Verification items for the finished model (mm, model axes). Face numbers are marked on the shaded views. A direction names the side the tool comes from. Give positions to 0.01 mm unless a question says otherwise; leave off trailing zeros. Loops run counter-clockwise (first coordinate to the right, second up) from the corner with the lowest first, then second, coordinate; pieces in that order, holes last. Notation, with made-up numbers: (71, -7.75) -> (117, -7.75) arc R15 cw to (117, 5.25) -> close; hole circle Ø6 at (61, -12). An arc over 180 degrees is marked (long way). Use one line per item in the form item = value. Start each with the question number.
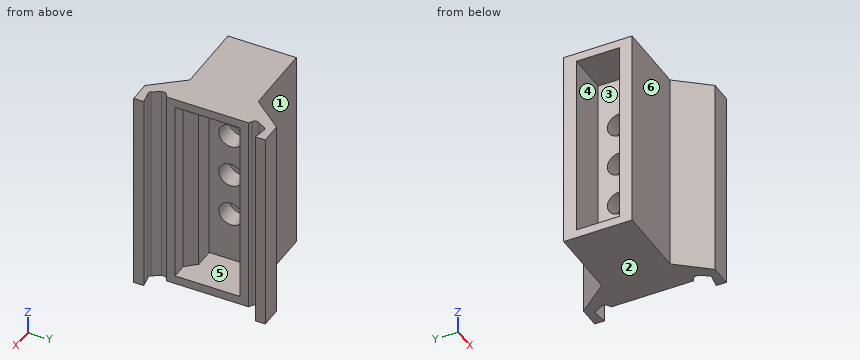
from build123d import *

# Parameters (mm, degrees)
BOSS_EXTRU_1_DEPTH      = 11.98
BOSS_EXTRU_1_DEPTH_BACK = 11.98
BOSS_EXTRU_2_DEPTH      = 1
ESQUISSE3_R             = 1.4
ENL_V_MAT_EXTRU_1_DEPTH = 16.868545408


with BuildPart() as part:
    # Esquisse1 → Boss.-Extru.1 (new, two sides: drawn at the far end of the back side and taken through both)
    with BuildSketch(Plane.XY.offset(-BOSS_EXTRU_1_DEPTH_BACK)):
        with BuildLine():
            Line((0, 4), (0, 2.5))
            Line((0, 2.5), (4.8, 2.5))
            Line((4.8, 2.5), (4.8, -2.5))
            Line((4.8, -2.5), (0, -2.5))
            Line((0, -2.5), (0, -4))
            Line((0, -4), (8.500076, -4))
            Line((8.500076, -4), (11.500006965, -7.699978353))
            Line((11.500006965, -7.699978353), (14, -7.699978353))
            Line((14, -7.699978353), (14, -6.524983133))
            Line((14, -6.524983133), (12.498521064, -6.789609096))
            ThreePointArc((12.498521064, -6.789609096), (12.319554673, -6.766083995), (12.186482634, -6.644124034))
            Line((12.186482634, -6.644124034), (11.641375242, -5.699594361))
            ThreePointArc((11.641375242, -5.699594361), (11.590815941, -5.322605229), (11.820116831, -5.019128457))
            Line((11.820116831, -5.019128457), (12.19995, -4.799870197))
            Line((12.19995, -4.799870197), (12.19995, -3.799987301))
            Line((12.19995, -3.799987301), (10.399918669, -3.799987301))
            Line((10.399918669, -3.799987301), (9.3, -2.549913972))
            Line((9.3, -2.549913972), (7, -2.549913972))
            Line((7, -2.549913972), (7, 2.550086028))
            Line((7, 2.550086028), (9.3, 2.550086028))
            Line((9.3, 2.550086028), (10.399918669, 3.800106202))
            Line((10.399918669, 3.800106202), (12.19995, 3.800106202))
            Line((12.19995, 3.800106202), (12.19995, 4.800033133))
            Line((12.19995, 4.800033133), (11.824382637, 5.01686254))
            ThreePointArc((11.824382637, 5.01686254), (11.591449393, 5.320453932), (11.641389736, 5.699837105))
            Line((11.641389736, 5.699837105), (12.186568343, 6.644209348))
            ThreePointArc((12.186568343, 6.644209348), (12.319573629, 6.766106706), (12.4984419, 6.789676051))
            Line((12.4984419, 6.789676051), (14, 6.524983133))
            Line((14, 6.524983133), (14, 7.700021647))
            Line((14, 7.700021647), (11.499988165, 7.700021647))
            Line((11.499988165, 7.700021647), (8.500082, 4))
            Line((8.500082, 4), (0, 4))
        make_face()
    extrude(amount=BOSS_EXTRU_1_DEPTH + BOSS_EXTRU_1_DEPTH_BACK)

    # Esquisse4 → Boss.-Extru.2 (add)
    with BuildSketch(Plane.XY.offset(11.98)):
        Polygon((10.399918669, 3.800106202), (12.19995, 3.800106202), (12.19995, -3.799987301), (10.399918669, -3.799987301), (9.3, -2.549913972), (7, -2.549913972), (0, -2.5), (0, 2.5), (7, 2.550086028), (9.3, 2.550086028), align=None)
    boss_extru_2 = extrude(amount=-BOSS_EXTRU_2_DEPTH)

    # Symétrie1: Boss.-Extru.2 across plane
    add(boss_extru_2.mirror(Plane.XY))

    # Esquisse3 → Enlèv. mat.-Extru.1 (cut, through all)
    with BuildSketch(Plane(origin=(7, 0, 0), x_dir=(0, 0, -1), z_dir=(1, 0, 0))):
        Circle(ESQUISSE3_R)
        with Locations((-5.08, 0)):
            Circle(ESQUISSE3_R)
        with Locations((5.08, 0)):
            Circle(ESQUISSE3_R)
    extrude(amount=-ENL_V_MAT_EXTRU_1_DEPTH, mode=Mode.SUBTRACT)


solid = part.part
Item 1: Draft check along Y on the marked faces 1, 2 and 3. Enter one of: +Y half, -Y half, draft (parallel to the pull), parting line (faces both ways), or undercut.
Item 2: Sectioned sample at A-A, the plane y = 0. Enter the section's corners in (x, z), and give its area (3 significant figures).
Item 3: Sectioned sample at B-B, the plane x = 6.5. Enter the section's corners in (y, z), and give its area (3 significant figures).
Item 4: Material ranges on line 1 (Y direction, x = 2.75, z = -8.25); line 2 (Y direction, x = 6.3, z = -5.08); line 3 (Z direction, x = 9, y = 0.5), recorded low to high.
Item 5: Gauge pin test, flat ends, axial feed: pin 1 Ø7 at (x, z) = (6, -5.5) entering from +Y; pin 2 Ø1.4 at (x, z) = (11, -2) entering from -Y; pin 3 Ø1.5 at (y, z) = (5, -7) entering from -X; pin 4 Ø1.8 at (x, z) = (8.5, 4.5) entering from -Y. Record the tip position at first contact, or that the pin passes through.
Item 6: Tool access check on the marked faces 4, 5 and 6. Record the directions out of +Z, -Z, +X, -X, +Y, -Y that give a thin tool (end or side, any length) a straight path to the whole face; none if there is none.
Item 7: Sectioned sample at D-D, the plane y = 2. Enter the section's corners in (x, z), and give its area (3 significant figures).
Outcome:
q1.face_1 = +Y half
q1.face_2 = draft
q1.face_3 = undercut
q2.outline = (0, -11.98) -> (12.2, -11.98) -> (12.2, -10.98) -> (7, -10.98) -> (7, -6.48) -> (4.8, -6.48) -> (4.8, -10.98) -> (0, -10.98) -> close; (0, 10.98) -> (4.8, 10.98) -> (4.8, 6.48) -> (7, 6.48) -> (7, 10.98) -> (12.2, 10.98) -> (12.2, 11.98) -> (0, 11.98) -> close; (4.8, -3.68) -> (7, -3.68) -> (7, -1.4) -> (4.8, -1.4) -> close; (4.8, 1.4) -> (7, 1.4) -> (7, 3.68) -> (4.8, 3.68) -> close
q2.area = 54.2 mm^2
q3.outline = (-4, -11.98) -> (4, -11.98) -> (4, 11.98) -> (-4, 11.98) -> close; hole circle Ø2.8 at (0, -5.08); hole circle Ø2.8 at (0, 0); hole circle Ø2.8 at (0, 5.08)
q3.area = 173 mm^2
q4.line_1 = -4 to -2.5, 2.5 to 4
q4.line_2 = -4 to -1.4, 1.4 to 4
q4.line_3 = -11.98 to -10.98, 10.98 to 11.98
q5.pin_1 = 5.23
q5.pin_2 = -7.7
q5.pin_3 = 8.7
q5.pin_4 = -5.11
q6.face_4 = -X
q6.face_5 = +X
q6.face_6 = +Z, -Z, -X, -Y
q7.outline = (0, -11.98) -> (12.2, -11.98) -> (12.2, -10.98) -> (7, -10.98) -> (7, 10.98) -> (12.2, 10.98) -> (12.2, 11.98) -> (0, 11.98) -> (0, 10.98) -> (4.8, 10.98) -> (4.8, -10.98) -> (0, -10.98) -> close
q7.area = 72.7 mm^2
